```python
from build123d import *

# Parameters (mm, degrees)
SKETCH_1_W          = 20
SKETCH_1_H          = 30
EXTRUDE_1_DEPTH     = 3.5
SKETCH_2_W          = 5.5
SKETCH_2_H          = 30
EXTRUDE_2_DEPTH     = 4.5
SKETCH_3_R          = 1.55
CUT_EXTRUDE_1_DEPTH = 8


with BuildPart() as part:
    # 草图1 → 凸台-拉伸1 (new body)
    with BuildSketch(Plane(origin=(0, 0, 0), x_dir=(1, 0, 0), z_dir=(0, 1, 0))):
        Rectangle(SKETCH_1_W, SKETCH_1_H)
    extrude(amount=EXTRUDE_1_DEPTH)

    # 草图2 → 凸台-拉伸2 (add)
    with BuildSketch(Plane(origin=(0, 0, 0), x_dir=(-1, 0, 0), z_dir=(0, -1, 0))):
        with Locations((-7.25, 0)):
            Rectangle(SKETCH_2_W, SKETCH_2_H)
        with Locations((7.25, 0)):
            Rectangle(SKETCH_2_W, SKETCH_2_H)
    extrude(amount=EXTRUDE_2_DEPTH)

    # 草图3 → 切除-拉伸1 (cut)
    with BuildSketch(Plane(origin=(0, 3.5, 0), x_dir=(1, 0, 0), z_dir=(0, 1, 0))):
        with Locations(Location((-7.5, -5, 0), (0, 0, 270))):
            Circle(SKETCH_3_R)
        with Locations(Location((-7.5, 5, 0), (0, 0, 270))):
            Circle(SKETCH_3_R)
        with Locations(Location((7.5, 5, 0), (0, 0, 270))):
            Circle(SKETCH_3_R)
        with Locations(Location((7.5, -5, 0), (0, 0, 270))):
            Circle(SKETCH_3_R)
    extrude(amount=-CUT_EXTRUDE_1_DEPTH, mode=Mode.SUBTRACT)


solid = part.part
```
The listing builds one solid part. Answer for the finished solid, in the listing's coordinates (mm). A direction names the side the tool comes from. Coordinates: 2 decimals unless noted, no trailing zeros. Loops run counter-clockwise (first coordinate to the right, second up) from the corner with the lowest first, then second, coordinate; pieces in that order, holes last. Notation, with made-up numbers: (23, 4) - (30, 4) arc R7 cw to (30, 9) - close; hole circle Ø11 at (40, 67). An arc over 180 degrees is marked (long way). Use a Markdown table: item, result. Add a question column.
1) The mould has two halves that part along Z. Classify faces 1 (the cylindrical face through (-8.44, -0.44, -6.23)), 2 (the flat face through (0, 3.5, 0)), 3 (the flat face through (0.1, 0.4, 15)): released by +Z, released by -Z, zero draft, split by the parting line, or undercut.
2) The part is cut by section B-B, the plane y = -2.5. Give the vertices of the cut face in (x, z).
3) The part is cut by section A-A, the plane z = -5. Give the vertices of the cut face in (x, y), and give its area (3 significant figures).
4) Find the intervals of material crossed by line 1 (X direction, y = 0.5, z = 5); line 2 (X direction, y = -3, z = -11); line 3 (X direction, y = -0.75, z = 5), in increasing order.
5) The part is cut by section C-C, the plane x = -7.5. Give the vertices of the cut face in (y, z).
6) The part is cut by section D-D, the plane y = 0.5. Give the vertices of the cut face in (x, z), and give its area (3 significant figures).
7) Given pin 1 (1.5 mm diameter, centred on x = 0.5, z = 10.5, fed in from -Y), flat-ended and moving along its own axis, determine where the tip first touches the part or whether it passes through.
8) For faces 4 (the flat face through (-10, -1, 0)), 5 (the flat face through (-4.5, -2, 0)), determine the directions among +Z, -Z, +X, -X, +Y, -Y from which every point of the face is accessible in a straight line to the end or side of a thin tool.
Here are the results:
| question | item | result |
|---|---|---|
| 1 | face 1 | undercut |
| 1 | face 2 | zero draft |
| 1 | face 3 | released by +Z |
| 2 | outline | (-10, -15) - (-4.5, -15) - (-4.5, 15) - (-10, 15) - close; (4.5, -15) - (10, -15) - (10, 15) - (4.5, 15) - close; hole circle Ø3.1 at (-7.5, -5); hole circle Ø3.1 at (-7.5, 5); hole circle Ø3.1 at (7.5, -5); hole circle Ø3.1 at (7.5, 5) |
| 3 | outline | (-10, -4.5) - (-9.05, -4.5) - (-9.05, 3.5) - (-10, 3.5) - close; (-5.95, -4.5) - (-4.5, -4.5) - (-4.5, 0) - (4.5, 0) - (4.5, -4.5) - (5.95, -4.5) - (5.95, 3.5) - (-5.95, 3.5) - close; (9.05, -4.5) - (10, -4.5) - (10, 3.5) - (9.05, 3.5) - close |
| 3 | area | 69.9 mm^2 |
| 4 | line 1 | x = -10 to -9.05, -5.95 to 5.95, 9.05 to 10 |
| 4 | line 2 | x = -10 to -4.5, 4.5 to 10 |
| 4 | line 3 | x = -10 to -9.05, -5.95 to -4.5, 4.5 to 5.95, 9.05 to 10 |
| 5 | outline | (-4.5, -15) - (3.5, -15) - (3.5, -6.55) - (-4.5, -6.55) - close; (-4.5, -3.45) - (3.5, -3.45) - (3.5, 3.45) - (-4.5, 3.45) - close; (-4.5, 6.55) - (3.5, 6.55) - (3.5, 15) - (-4.5, 15) - close |
| 6 | outline | (-10, -15) - (10, -15) - (10, 15) - (-10, 15) - close; hole circle Ø3.1 at (-7.5, -5); hole circle Ø3.1 at (-7.5, 5); hole circle Ø3.1 at (7.5, -5); hole circle Ø3.1 at (7.5, 5) |
| 6 | area | 570 mm^2 |
| 7 | pin 1 | stops at y = 0 |
| 8 | face 4 | +Z, -Z, -X, +Y, -Y |
| 8 | face 5 | +Z, -Z, -Y |
